Can you work these out from the model? Positions are in its coordinate system, mm. A direction names the side the tool comes from. Give positions to 0.01 mm unless a question says otherwise; leave off trailing zeros. Loops run counter-clockwise (first coordinate to the right, second up) from the corner with the lowest first, then second, coordinate; pieces in that order, holes last.
from build123d import *

# Parameters (mm, degrees)
CYLINDER1792_R         = 35
CYLINDER1792_DEPTH     = 32
CYLINDER1789_R         = 3
CYLINDER1789_DEPTH     = 3
CYLINDER1790_R         = 3
CYLINDER1790_DEPTH     = 3
CYLINDER1791_R         = 3
CYLINDER1791_DEPTH     = 3
CYLINDER1788_R         = 3
CYLINDER1788_DEPTH     = 3
CYLINDER1785_R         = 1.5
CYLINDER1785_DEPTH     = 60
CYLINDER1786_R         = 1.5
CYLINDER1786_DEPTH     = 60
CYLINDER1787_R         = 1.5
CYLINDER1787_DEPTH     = 60
CYLINDER1784_R         = 1.5
CYLINDER1784_DEPTH     = 60
BOX710_W               = 42
BOX710_H               = 64
BOX710_DEPTH           = 50
BOX709_W               = 54
BOX709_H               = 68
BOX709_DEPTH           = 9
CHAMFER059_SIZE        = 3
CHAMFER060_SIZE        = 2
CHAMFER061_SIZE        = 1
CUT521_PLACEMENT_ANGLE = 90
CUT525_PLACEMENT_ANGLE = 180


with BuildPart() as obj1:
    # Cylinder1792 → Cylinder1792 (new body)
    with BuildSketch(Plane.XY.offset(-3)):
        Circle(CYLINDER1792_R)
    extrude(amount=CYLINDER1792_DEPTH)


with BuildPart() as obj2:
    # Cylinder1789 → Cylinder1789 (new body)
    with BuildSketch(Plane(origin=(-24, 73, -80), x_dir=(1, 0, 0), z_dir=(0, 0, 1))):
        Circle(CYLINDER1789_R)
    extrude(amount=CYLINDER1789_DEPTH)


with BuildPart() as obj3:
    # Cylinder1790 → Cylinder1790 (new body)
    with BuildSketch(Plane(origin=(-15, 125, -80), x_dir=(1, 0, 0), z_dir=(0, 0, 1))):
        Circle(CYLINDER1790_R)
    extrude(amount=CYLINDER1790_DEPTH)


with BuildPart() as obj4:
    # Cylinder1791 → Cylinder1791 (new body)
    with BuildSketch(Plane(origin=(15, 125, -80), x_dir=(1, 0, 0), z_dir=(0, 0, 1))):
        Circle(CYLINDER1791_R)
    extrude(amount=CYLINDER1791_DEPTH)


with BuildPart() as compound888:
    # Cylinder1788 → Cylinder1788 (new body)
    with BuildSketch(Plane(origin=(24, 73, -80), x_dir=(1, 0, 0), z_dir=(0, 0, 1))):
        Circle(CYLINDER1788_R)
    extrude(amount=CYLINDER1788_DEPTH)

    # Compound888: union obj2, obj3, obj4
    add(obj2.part)
    add(obj3.part)
    add(obj4.part)


with BuildPart() as compound888_1:
    # Compound888 placement: moved
    add(compound888.part.moved(Location((0, 0, 161))))


with BuildPart() as obj5:
    # Cylinder1785 → Cylinder1785 (new body)
    with BuildSketch(Plane(origin=(-24, 73, -80), x_dir=(1, 0, 0), z_dir=(0, 0, 1))):
        Circle(CYLINDER1785_R)
    extrude(amount=CYLINDER1785_DEPTH)


with BuildPart() as obj6:
    # Cylinder1786 → Cylinder1786 (new body)
    with BuildSketch(Plane(origin=(-15, 125, -80), x_dir=(1, 0, 0), z_dir=(0, 0, 1))):
        Circle(CYLINDER1786_R)
    extrude(amount=CYLINDER1786_DEPTH)


with BuildPart() as obj7:
    # Cylinder1787 → Cylinder1787 (new body)
    with BuildSketch(Plane(origin=(15, 125, -80), x_dir=(1, 0, 0), z_dir=(0, 0, 1))):
        Circle(CYLINDER1787_R)
    extrude(amount=CYLINDER1787_DEPTH)


with BuildPart() as compound887:
    # Cylinder1784 → Cylinder1784 (new body)
    with BuildSketch(Plane(origin=(24, 73, -80), x_dir=(1, 0, 0), z_dir=(0, 0, 1))):
        Circle(CYLINDER1784_R)
    extrude(amount=CYLINDER1784_DEPTH)

    # Compound887: union obj5, obj6, obj7
    add(obj5.part)
    add(obj6.part)
    add(obj7.part)


with BuildPart() as compound887_1:
    # Compound887 placement: moved
    add(compound887.part.moved(Location((0, 0, 120))))


with BuildPart() as krychle710:
    # Box710 → Box710 (new body)
    with BuildSketch(Plane(origin=(-21, 58, 38), x_dir=(1, 0, 0), z_dir=(0, 0, 1))):
        with Locations((21, 32)):
            Rectangle(BOX710_W, BOX710_H)
    extrude(amount=BOX710_DEPTH)


with BuildPart() as cut525:
    # Box709 → Box709 (new body)
    with BuildSketch(Plane(origin=(-27.004408, 59.99801, 75), x_dir=(1, 0, 0), z_dir=(0, 0, 1))):
        with Locations((27, 34)):
            Rectangle(BOX709_W, BOX709_H)
    extrude(amount=BOX709_DEPTH)

    # Cut519: cut Krychle710
    add(krychle710.part, mode=Mode.SUBTRACT)

    # Chamfer059
    chamfer059_edges = [cut525.edges().sort_by_distance(p)[0] for p in [
        (-27.004408, 127.99801, 79.5),
        (26.995592, 127.99801, 79.5),
    ]]
    chamfer(chamfer059_edges, length=CHAMFER059_SIZE)

    # Chamfer060
    chamfer060_edges = [cut525.edges().sort_by_distance(p)[0] for p in [
        (-27.004408, 92.49801, 84),
        (26.995592, 92.49801, 84),
    ]]
    chamfer(chamfer060_edges, length=CHAMFER060_SIZE)

    # Chamfer061
    chamfer061_edges = [cut525.edges().sort_by_distance(p)[0] for p in [
        (-0.004408, 127.99801, 84),
    ]]
    chamfer(chamfer061_edges, length=CHAMFER061_SIZE)

    # Cut520: cut Compound887
    add(compound887_1.part, mode=Mode.SUBTRACT)

    # Cut521: cut Compound888
    add(compound888_1.part, mode=Mode.SUBTRACT)


with BuildPart() as cut525_1:
    # Cut521 placement: moved
    add(cut525.part.moved(Location((-39, 0, -59))).rotate(Axis((-39, 0, -59), (0, 0, -1)), CUT521_PLACEMENT_ANGLE))

    # Cut525: cut obj1
    add(obj1.part, mode=Mode.SUBTRACT)


with BuildPart() as cut525_2:
    # Cut525 placement: moved
    add(cut525_1.part.rotate(Axis((0, 0, 0), (0, 0, 1)), CUT525_PLACEMENT_ANGLE))


solid = cut525_2.part
(1) Suppose I cut it at B-B on z = 19.5. List the corners of the cut face in (x, y) for me, plus the area to 3 significant figures.
Returned:
outline: (-89, -24) - (-86, -27) - (-22.27, -27) arc R35 cw to (-28, -21) - (-83, -21) - (-83, 21) - (-28, 21) arc R35 cw to (-22.28, 27) - (-86, 27) - (-89, 24) - close; hole circle Ø3 at (-86, -15); hole circle Ø3 at (-86, 15); hole circle Ø3 at (-34, -24); hole circle Ø3 at (-34, 24)
area: 978 mm2
(2) Suppose I cut it at C-C on y = -7. List the corners of the cut face in (x, z) for me, plus the area to 3 significant figures.
Returned:
outline: (-89, 16) - (-83, 16) - (-83, 25) - (-88, 25) - (-89, 24) - close
area: 53.5 mm2
(3) Thinking about a two-plate mould opening in X: for faces 1 (the flat face through (-29, -23, 25)), 2 (the cylindrical face through (-25.276, 24.21, 20.437)), 3 (the cylindrical face through (-86, 12, 23)), which applies, pulls with the +X half, pulls with the -X half, needs draft (parallel to the pull), parting line crosses it, or undercut?
Returned:
face 1: needs draft
face 2: pulls with the +X half
face 3: undercut
(4) Please list where these lines run through material, in increasing order: probe 1 along Y at (x, z) = (-86, 20); probe 2 along Y at (x, z) = (-34, 20); probe 3 along Y at (x, z) = (-50, 17.5).
Returned:
probe 1: y = -27 to -16.5, -13.5 to 13.5, 16.5 to 26.99
probe 2: y = -27 to -25.5, -22.5 to -21, 21 to 22.5, 25.5 to 27
probe 3: y = -27 to -21, 21 to 27
(5) Suppose I cut it at A-A on x = -77. List the corners of the cut face in (y, z) for me.
Returned:
outline: (-27, 16) - (-21, 16) - (-21, 25) - (-25, 25) - (-27, 23) - close; (21, 16) - (27, 16) - (27, 23) - (25, 25) - (21, 25) - close
(6) Which directions (+Z, -Z, +X, -X, +Y, -Y) give clear straight access to the entire face, cutting with the end or side of a thin tool? Please do faces 4 (the cylindrical face through (-86, -12, 23)), 5 (the flat face through (-54.672, -25.99, 24.014)), 6 (the flat face through (-55, -21, 20)).
Returned:
face 4: +Z
face 5: +Z, +X, -X, -Y
face 6: +Z, -Z, +X
(7) Will these pins go through, and if not, where does the flat tip stop? P1, Ø3, axis at x = -35, y = -24, coming from the +Z side; P2, Ø2, axis at y = 11, z = 23, coming from the +X side; P3, Ø1.5, axis at x = -79, z = 23.5, coming from the +Y side.
Returned:
P1: stops at z = 22
P2: stops at x = -83
P3: stops at y = 27
